Could you check a few things on this drawing? It's one solid part, dimensions in mm from its lowest x, y, z. Round coordinates to 2 decimals unless told otherwise and drop trailing zeros. Order: outer loops, then holes, each group sorted by start corner. A loop starts at its lowest first (then second) coordinate and runs counter-clockwise, first axis right, second up.
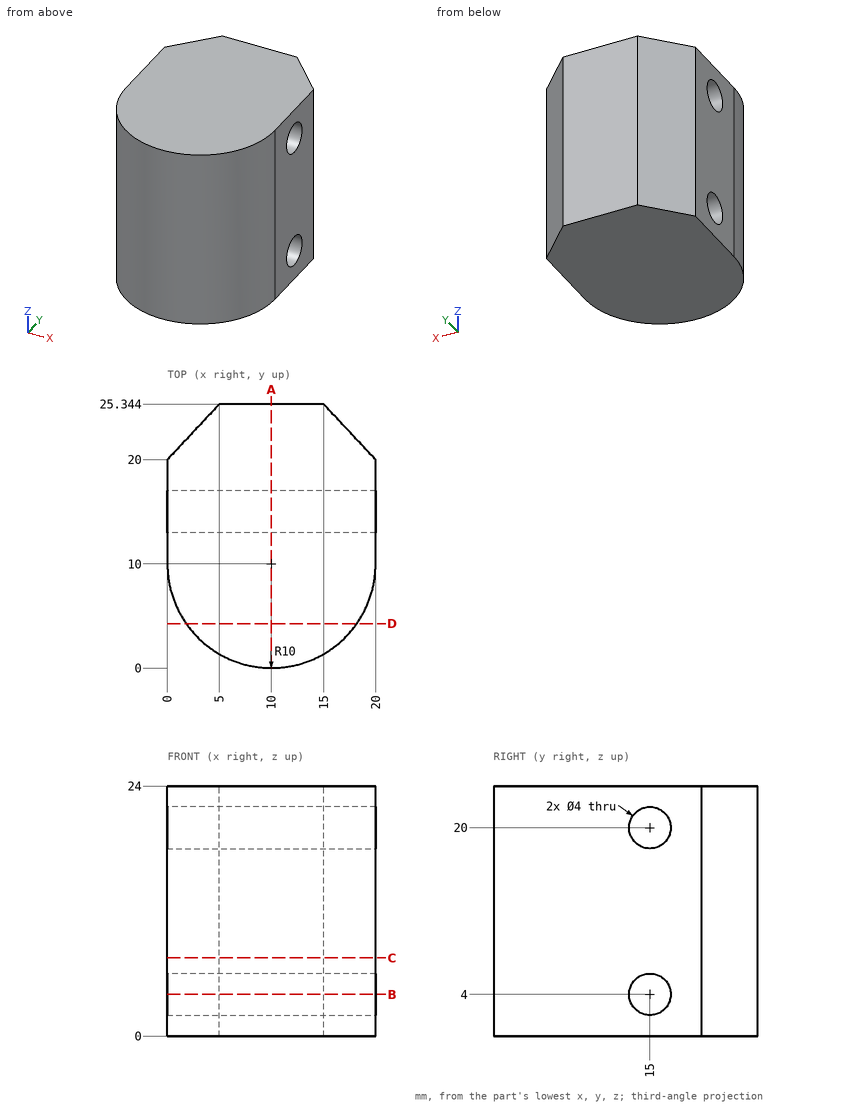
(1) I want a section at A-A, the plane x = 10. List the corners of the cut face in (y, z) for me (1 decimal), plus the area to 3 significant figures.
(2) I want a section at D-D, the plane y = 4.25. List the corners of the cut face in (x, z) for me.
(3) I'm going to push a flat-ended pin straight in: pin 1 Ø1.5 at (y, z) = (16, 20.5) entering from +X. Where does the tip first touch, or does it pass through?
(4) I want a section at B-B, the plane z = 4. List the corners of the cut face in (x, y) for me (1 decimal), plus the area to 3 significant figures.
(5) Please list where these lines run through material, in increasing order: probe 1 along Z at (x, y) = (9.5, 15); probe 2 along Y at (x, z) = (14.5, 20) (1 decimal); probe 3 along Y at (x, z) = (4, 20) (1 decimal).
(6) I want a section at C-C, the plane z = 7.5. List the corners of the cut face in (x, y) for me (1 decimal).
Ans:
1. outline: (0, 0) - (25.3, 0) - (25.3, 24) - (0, 24) - close; hole circle Ø4 at (15, 4); hole circle Ø4 at (15, 20)
1. area: 583 mm2
2. outline: (1.82, 0) - (18.18, 0) - (18.18, 24) - (1.82, 24) - close
3. pin 1: passes through
4. outline: (0, 10) arc R10 ccw to (20, 10) - (20, 13) - (0, 13) - close; (0, 17) - (20, 17) - (20, 20) - (15, 25.3) - (5, 25.3) - (0, 20) - close
4. area: 357 mm2
5. probe 1: z = 0 to 2, 6 to 18, 22 to 24
5. probe 2: y = 1.1 to 13, 17 to 25.3
5. probe 3: y = 2 to 13, 17 to 24.3
6. outline: (0, 10) arc R10 ccw to (20, 10) - (20, 20) - (15, 25.3) - (5, 25.3) - (0, 20) - close
